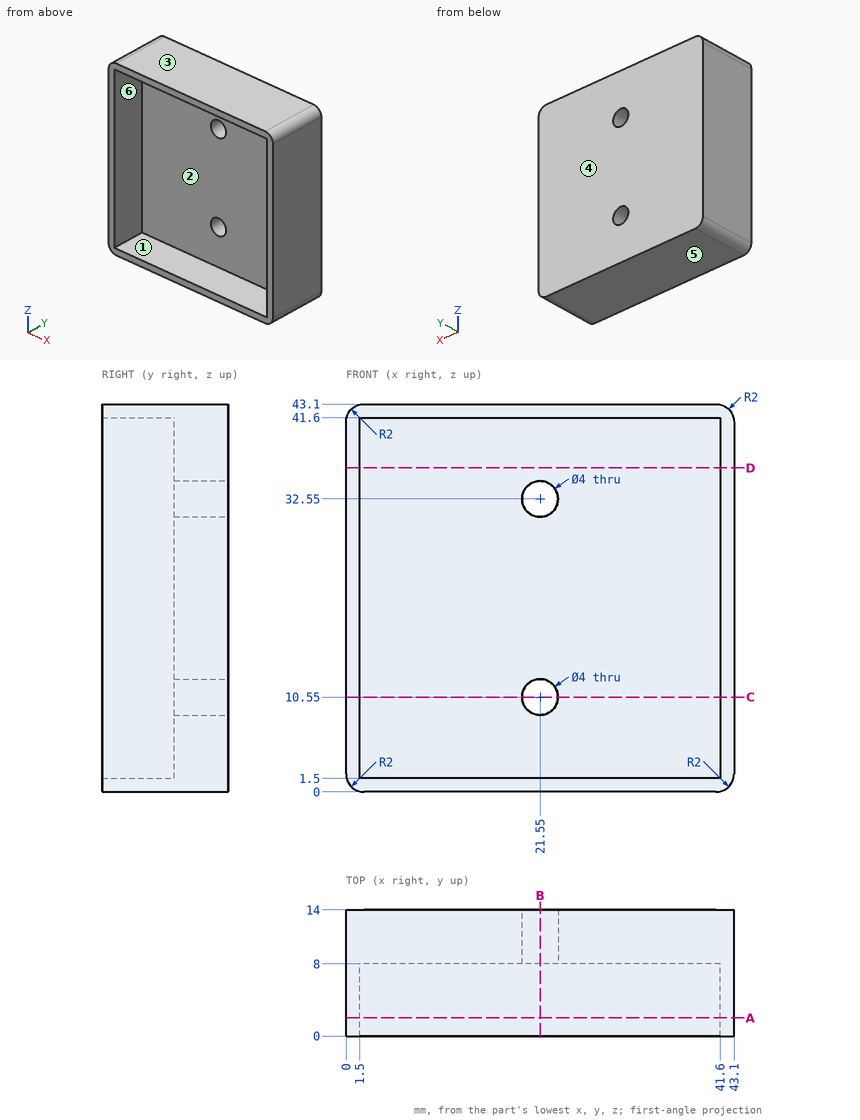
The drawing under review shows one solid part. Ordinate dimensions are in mm from its lowest x, y, z. A direction names the side the tool comes from. Give positions to 0.01 mm unless a question says otherwise; leave off trailing zeros. Write each loop counter-clockwise with the first axis right and the second up, starting at its lowest first coordinate (ties: lowest second). Pieces come first, ordered by that corner, then holes. Notation, with made-up numbers: (41.25, 46) -> (51.25, 46) arc R23 ccw to (51.25, 84) -> close; hole circle Ø11 at (-2, 13). An arc over 180 degrees is marked (long way). Use CSV: the item, a comma, the result in double quotes.
Q1. Take a section at A-A, the plane y = 2. Write out the cut boundary in (x, z).
Conclusion:
outline,"(0, 2) arc R2 ccw to (2, 0) -> (41.1, 0) arc R2 ccw to (43.1, 2) -> (43.1, 41.1) arc R2 ccw to (41.1, 43.1) -> (2, 43.1) arc R2 ccw to (0, 41.1) -> close; hole (1.5, 1.5) -> (41.6, 1.5) -> (41.6, 41.6) -> (1.5, 41.6) -> close"
Q2. Tool access review of the marked faces 5 and 6: name each direction out of +Z, -Z, +X, -X, +Y, -Y from which nothing blocks a thin tool from reaching the whole face with its end or side.
Conclusion:
face 5,"-Z, +X, -X, +Y, -Y"
face 6,"-Y"
Q3. Take a section at D-D, the plane z = 36. Write out the cut boundary in (x, y), then the cut area to 3 significant figures.
Conclusion:
outline,"(0, 0) -> (1.5, 0) -> (1.5, 8) -> (41.6, 8) -> (41.6, 0) -> (43.1, 0) -> (43.1, 14) -> (0, 14) -> close"
area,"283 mm2"
Q4. Take a section at C-C, the plane z = 10.55. Write out the cut boundary in (x, y).
Conclusion:
outline,"(0, 0) -> (1.5, 0) -> (1.5, 8) -> (19.55, 8) -> (19.55, 14) -> (0, 14) -> close; (23.55, 8) -> (41.6, 8) -> (41.6, 0) -> (43.1, 0) -> (43.1, 14) -> (23.55, 14) -> close"
Q5. To check wall thickness, follow probe 1 along Z at (x, y) = (21.55, 10.75); probe 2 along X at (y, z) = (6.5, 19); probe 3 along X at (y, z) = (12.25, 32.55). State the ranges of each line that lie inside material, in increasing order. Write a range as [from, to].
Conclusion:
probe 1,"[0, 8.55], [12.55, 30.55], [34.55, 43.1]"
probe 2,"[0, 1.5], [41.6, 43.1]"
probe 3,"[0, 19.55], [23.55, 43.1]"
Q6. For P1, Ø3.5, axis at x = 21.55, z = 32.55, coming from the +Y side; P2, Ø1, axis at x = 26.5, z = 36.5, coming from the -Y side; P3, Ø6.5, axis at x = 22, y = 2.5, coming from the -Z side, all flat-tipped, find the tip position at first contact; note any pin that passes through.
Conclusion:
P1,"through"
P2,"y = 8"
P3,"z = 0"
Q7. Mouldability with a two-part tool opening along Z and no side actions: class the marked faces 1, 2, 3 and 4 as pulls with the +Z half, pulls with the -Z half, needs draft (parallel to the pull), parting line crosses it, or undercut.
Conclusion:
face 1,"undercut"
face 2,"undercut"
face 3,"pulls with the +Z half"
face 4,"needs draft"
Q8. Take a section at B-B, the plane x = 21.55. Write out the cut boundary in (y, z).
Conclusion:
outline,"(0, 0) -> (14, 0) -> (14, 8.55) -> (8, 8.55) -> (8, 1.5) -> (0, 1.5) -> close; (0, 41.6) -> (8, 41.6) -> (8, 34.55) -> (14, 34.55) -> (14, 43.1) -> (0, 43.1) -> close; (8, 12.55) -> (14, 12.55) -> (14, 30.55) -> (8, 30.55) -> close"
